Geometry check sheet. Reference: the model listing, model coordinates, mm. Face numbers are marked on the shaded views. A direction names the side the tool comes from. Coordinates: 2 decimals unless noted, no trailing zeros. Loops run counter-clockwise (first coordinate to the right, second up) from the corner with the lowest first, then second, coordinate; pieces in that order, holes last.
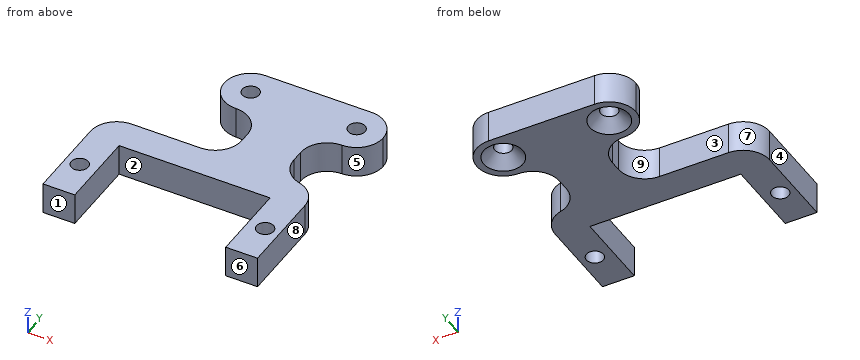
from build123d import *

# Parameters (mm, degrees)
BOSS_EXTRU_1_DEPTH      = 6
ESQUISSE2_R             = 1.6
ENL_V_MAT_EXTRU_1_DEPTH = 10
ESQUISSE4_R             = 1.6
ENL_V_MAT_EXTRU_2_DEPTH = 37.572701568
CHANFREIN1_SIZE         = 2.1
CONG_1_R                = 5
CONG_2_R                = 5


with BuildPart() as part:
    # Esquisse1 → Boss.-Extru.1 (new body)
    with BuildSketch(Plane.XY):
        Polygon((12.75, 18), (22.75, 18), (22.75, 28), (-7.25, 28), (-7.25, 18), (2.75, 18), (2.75, 6), (-20.25, 6), (-20.25, 0), (-20.25, -15), (-14.25, -15), (-14.25, 0), (14.25, 0), (14.25, -15), (20.25, -15), (20.25, -0.694767442), (20.25, 6), (12.75, 6), align=None)
    extrude(amount=BOSS_EXTRU_1_DEPTH)

    # Esquisse2 → Enlèv. mat.-Extru.1 (cut)
    with BuildSketch(Plane.XY.offset(6)):
        with Locations((-17.5, -7.5)):
            Circle(ESQUISSE2_R)
        with Locations((17.5, -7.5)):
            Circle(ESQUISSE2_R)
    extrude(amount=-ENL_V_MAT_EXTRU_1_DEPTH, mode=Mode.SUBTRACT)

    # Esquisse4 → Enlèv. mat.-Extru.2 (cut, through all)
    with BuildSketch(Plane(origin=(0, 0, 0), x_dir=(-1, 0, 0), z_dir=(0, 0, -1))):
        with Locations((-17.75, 23)):
            Circle(ESQUISSE4_R)
        with Locations((2.25, 23)):
            Circle(ESQUISSE4_R)
    extrude(amount=-ENL_V_MAT_EXTRU_2_DEPTH, mode=Mode.SUBTRACT)

    # Chanfrein1
    chanfrein1_edges = [part.edges().sort_by_distance(p)[0] for p in [
        (19.35, 23, 0),
        (-0.65, 23, 0),
    ]]
    chamfer(chanfrein1_edges, length=CHANFREIN1_SIZE)

    # Congé1
    cong_1_edges = [part.edges().sort_by_distance(p)[0] for p in [
        (2.75, 6, 3),
        (-20.25, 6, 3),
        (20.25, 6, 3),
        (-7.25, 28, 3),
        (-7.25, 18, 3),
        (2.75, 18, 3),
        (12.75, 18, 3),
        (22.75, 18, 3),
        (22.75, 28, 3),
    ]]
    fillet(cong_1_edges, radius=CONG_1_R - 0.0001)  # a hair under: the kernel refuses the full size

    # Congé2
    cong_2_edges = [part.edges().sort_by_distance(p)[0] for p in [
        (12.75, 6, 3),
    ]]
    fillet(cong_2_edges, radius=CONG_2_R)


solid = part.part
1) Access from +Z, -Z, +X, -X, +Y, -Y to the whole of each face (thin tool, end or side, straight path). Record for the marked faces 1, 2, 3, 4 and 5.
Data:
face 1: +Z, -Z, +X, -X, -Y
face 2: +Z, -Z, -Y
face 3: +Z, -Z, -X
face 4: +Z, -Z, -X, +Y, -Y
face 5: +Z, -Z, +X
2) Section check D-D on x = -9. Record the cut outline in (y, z).
Data:
outline: (0, 0) - (6, 0) - (6, 6) - (0, 6) - close
3) Section check A-A on y = -7.5. Record the cut outline in (x, z), and give its area (3 significant figures).
Data:
outline: (-20.25, 0) - (-19.1, 0) - (-19.1, 6) - (-20.25, 6) - close; (-15.9, 0) - (-14.25, 0) - (-14.25, 6) - (-15.9, 6) - close; (14.25, 0) - (15.9, 0) - (15.9, 6) - (14.25, 6) - close; (19.1, 0) - (20.25, 0) - (20.25, 6) - (19.1, 6) - close
area: 33.6 mm2
4) Section check C-C on z = 0.75. Count the separate pieces of the cut face and the enclosed holes in it, and give its area (3 significant figures).
Data:
separate pieces: 1
enclosed holes: 4
area: 760 mm2
5) Depth check by flat-ended pin: pin 1 (0.6 mm diameter, centred on y = 11.5, z = 4.5, fed in from -X); pin 2 (2 mm diameter, centred on y = 4, z = 2, fed in from +X); pin 3 (1.5 mm diameter, centred on y = -10, z = 5, fed in from +X); pin 4 (3 mm diameter, centred on x = -17.5, y = -7.5, fed in from +Z). Enter the tip coordinate at first touch or a pass-through.
Data:
pin 1: stops at x = 2.75
pin 2: stops at x = 19.83
pin 3: stops at x = 20.25
pin 4: passes through
6) Mould release check, pull along Y, two halves, no side actions. Record for the marked faces 6, 7, 8 and 9: +Y half, -Y half, draft (parallel to the pull), parting line (faces both ways), or undercut.
Data:
face 6: -Y half
face 7: +Y half
face 8: draft
face 9: undercut
7) Section check B-B on x = -17.5. Record the cut outline in (y, z), and give its area (3 significant figures).
Data:
outline: (-15, 0) - (-9.1, 0) - (-9.1, 6) - (-15, 6) - close; (-5.9, 0) - (5.47, 0) - (5.47, 6) - (-5.9, 6) - close
area: 104 mm2
8) Material ranges on probe 1 along Y at (x, z) = (-2.25, 3.9); probe 2 along Y at (x, z) = (17.5, 4.55); probe 3 along X at (y, z) = (11, 1.25), recorded low to high.
Data:
probe 1: y = 0 to 6, 18 to 21.4, 24.6 to 28
probe 2: y = -15 to -9.1, -5.9 to 5.47, 17.99 to 21.42, 24.58 to 28
probe 3: x = 2.75 to 12.75
